Could you check a few things on this model? Use its own coordinates, in mm. Give positions to 0.01 mm unless a question says otherwise; leave off trailing zeros. Loops run counter-clockwise (first coordinate to the right, second up) from the corner with the lowest first, then second, coordinate; pieces in that order, holes last. Notation, with made-up numbers: M -33.75,-3.75 L 15.25,-3.75 A24 ccw 15.25,21.25 Z; hole C 47,14 d3. An arc over 180 degrees is marked long. Return JSON: item names as keys, results as strings. Group by question number.
1. If we section it at C-C (x = 3.83): Write out the boundary of the cut face in (y, z).
2. If we section it at B-B (x = 44.17): State how many separate pieces and enclosed holes the cut face has, plus the area to 3 significant figures.
3. Please list where these lines run through material, in increasing order: line 1 (Y direction, x = -44.17, z = 0.9) (3 decimals); line 2 (X direction, y = 120, z = 0.05); line 3 (X direction, y = 132, z = -0.7).
4. If we section it at D-D (y = 140): Write out the boundary of the cut face in (x, z).
5. If we section it at A-A (y = 90): Write out the boundary of the cut face in (x, z).
6. For pin 1 (4 mm diameter, centred on x = 44.17, y = 120, fed in from -Z), with a flat end and sliding along its axis, tell me the tip position at first contact or that it passes through.
```python
from build123d import *

# Parameters (mm, degrees)
STOCK_TORSO_REAR_PLATE_1_START       = -1.5875
STOCK_TORSO_REAR_PLATE_1_OUTLINE_W   = 96.34
STOCK_TORSO_REAR_PLATE_1_OUTLINE_H   = 125.5
STOCK_TORSO_REAR_PLATE_1_OUTLINE_R   = 1.45
STOCK_TORSO_REAR_PLATE_1_OUTLINE_W_2 = 3.4925
STOCK_TORSO_REAR_PLATE_1_OUTLINE_H_2 = 10.25
STOCK_TORSO_REAR_PLATE_1_DEPTH       = 3.175
MOVE_FACE1_BY                        = 0.5
CUT_EXTRUDE1_DEPTH                   = 158.576741701
CUT_EXTRUDE1_DEPTH_BACK              = 158.576741701
CUT_EXTRUDE2_DEPTH                   = 158.576741701
CUT_EXTRUDE2_DEPTH_BACK              = 158.576741701
SKETCH2_W                            = 25
SKETCH2_H                            = 62
FILLET1_R                            = 1
CUT_EXTRUDE3_DEPTH                   = 158.576741701
CUT_EXTRUDE3_DEPTH_BACK              = 158.576741701
FILLET2_R                            = 1


# Read off the part's stored shape, not the designer's step: Stock-torso_rear_plate-1
with BuildPart() as part:
    # Stock-torso_rear_plate-1 outline → Stock-torso_rear_plate-1 (new body)
    with BuildSketch(Plane.XY.offset(STOCK_TORSO_REAR_PLATE_1_START)):
        with Locations((0, 87.25)):
            Rectangle(STOCK_TORSO_REAR_PLATE_1_OUTLINE_W, STOCK_TORSO_REAR_PLATE_1_OUTLINE_H)
        with Locations((-44.17, 40)):
            Circle(STOCK_TORSO_REAR_PLATE_1_OUTLINE_R, mode=Mode.SUBTRACT)
        with BuildLine():
            Line((30, 34.5), (-30, 34.5))
            ThreePointArc((-30, 34.5), (-32.5, 37), (-30, 39.5))
            Line((-30, 39.5), (30, 39.5))
            ThreePointArc((30, 39.5), (32.5, 37), (30, 34.5))
        make_face(mode=Mode.SUBTRACT)
        with BuildLine():
            Line((30, 44.5), (-30, 44.5))
            ThreePointArc((-30, 44.5), (-32.5, 47), (-30, 49.5))
            Line((-30, 49.5), (30, 49.5))
            ThreePointArc((30, 49.5), (32.5, 47), (30, 44.5))
        make_face(mode=Mode.SUBTRACT)
        with Locations((44.17, 40)):
            Circle(STOCK_TORSO_REAR_PLATE_1_OUTLINE_R, mode=Mode.SUBTRACT)
        with BuildLine():
            ThreePointArc((-30, 54.5), (-32.5, 57), (-30, 59.5))
            Line((-30, 59.5), (30, 59.5))
            ThreePointArc((30, 59.5), (32.5, 57), (30, 54.5))
            Line((30, 54.5), (-30, 54.5))
        make_face(mode=Mode.SUBTRACT)
        with BuildLine():
            ThreePointArc((-30, 64.5), (-32.5, 67), (-30, 69.5))
            Line((-30, 69.5), (30, 69.5))
            ThreePointArc((30, 69.5), (32.5, 67), (30, 64.5))
            Line((30, 64.5), (-30, 64.5))
        make_face(mode=Mode.SUBTRACT)
        with Locations((-44.17, 120)):
            Circle(STOCK_TORSO_REAR_PLATE_1_OUTLINE_R, mode=Mode.SUBTRACT)
        with Locations((-44.17, 141)):
            Rectangle(STOCK_TORSO_REAR_PLATE_1_OUTLINE_W_2, STOCK_TORSO_REAR_PLATE_1_OUTLINE_H_2, mode=Mode.SUBTRACT)
        with Locations((44.17, 120)):
            Circle(STOCK_TORSO_REAR_PLATE_1_OUTLINE_R, mode=Mode.SUBTRACT)
        with Locations((44.17, 141)):
            Rectangle(STOCK_TORSO_REAR_PLATE_1_OUTLINE_W_2, STOCK_TORSO_REAR_PLATE_1_OUTLINE_H_2, mode=Mode.SUBTRACT)
    extrude(amount=STOCK_TORSO_REAR_PLATE_1_DEPTH)

    # Move Face1: a face moved inward by 0.5
    extrude(part.faces().sort_by_distance((0, 24.5, 0))[0], amount=MOVE_FACE1_BY, dir=(0, 1, 0), mode=Mode.SUBTRACT)

    # Sketch1 → Cut-Extrude1 (cut, two sides: drawn at the far end of the back side and taken through both)
    with BuildSketch(Plane.XY.offset(1.5875).offset(-CUT_EXTRUDE1_DEPTH_BACK)):
        with BuildLine():
            Line((1.83, 75), (1.83, 79))
            ThreePointArc((1.83, 79), (3.83, 81), (5.83, 79))
            Line((5.83, 79), (5.83, 75))
            ThreePointArc((5.83, 75), (3.83, 73), (1.83, 75))
        make_face()
        with BuildLine():
            Line((16.83, 75), (16.83, 79))
            ThreePointArc((16.83, 79), (18.83, 81), (20.83, 79))
            Line((20.83, 79), (20.83, 75))
            ThreePointArc((20.83, 75), (18.83, 73), (16.83, 75))
        make_face()
    extrude(amount=CUT_EXTRUDE1_DEPTH + CUT_EXTRUDE1_DEPTH_BACK, mode=Mode.SUBTRACT)

    # Sketch2 → Cut-Extrude2 (cut, two sides: drawn at the far end of the back side and taken through both)
    with BuildSketch(Plane(origin=(0, 0, -1.5875), x_dir=(-1, 0, 0), z_dir=(0, 0, -1)).offset(-CUT_EXTRUDE2_DEPTH_BACK)):
        with Locations((-23.67, 114)):
            Rectangle(SKETCH2_W, SKETCH2_H)
    extrude(amount=CUT_EXTRUDE2_DEPTH + CUT_EXTRUDE2_DEPTH_BACK, mode=Mode.SUBTRACT)

    # Fillet1
    fillet1_edges = [part.edges().sort_by_distance(p)[0] for p in [
        (36.17, 83, 0),
        (36.17, 145, 0),
        (11.17, 145, 0),
        (11.17, 83, 0),
    ]]
    fillet(fillet1_edges, radius=FILLET1_R)

    # Sketch3 → Cut-Extrude3 (cut, two sides: drawn at the far end of the back side and taken through both)
    with BuildSketch(Plane(origin=(0, 0, -1.5875), x_dir=(-1, 0, 0), z_dir=(0, 0, -1)).offset(-CUT_EXTRUDE3_DEPTH_BACK)):
        with BuildLine():
            Line((0, 92.5), (30, 92.5))
            ThreePointArc((30, 92.5), (32.5, 90), (30, 87.5))
            Line((30, 87.5), (0, 87.5))
            ThreePointArc((0, 87.5), (-2.5, 90), (0, 92.5))
        make_face()
        with BuildLine():
            Line((0, 102.5), (30, 102.5))
            ThreePointArc((30, 102.5), (32.5, 100), (30, 97.5))
            Line((30, 97.5), (0, 97.5))
            ThreePointArc((0, 97.5), (-2.5, 100), (0, 102.5))
        make_face()
        with BuildLine():
            Line((0, 112.5), (30, 112.5))
            ThreePointArc((30, 112.5), (32.5, 110), (30, 107.5))
            Line((30, 107.5), (0, 107.5))
            ThreePointArc((0, 107.5), (-2.5, 110), (0, 112.5))
        make_face()
        with BuildLine():
            Line((0, 122.5), (30, 122.5))
            ThreePointArc((30, 122.5), (32.5, 120), (30, 117.5))
            Line((30, 117.5), (0, 117.5))
            ThreePointArc((0, 117.5), (-2.5, 120), (0, 122.5))
        make_face()
        with BuildLine():
            Line((0, 132.5), (30, 132.5))
            ThreePointArc((30, 132.5), (32.5, 130), (30, 127.5))
            Line((30, 127.5), (0, 127.5))
            ThreePointArc((0, 127.5), (-2.5, 130), (0, 132.5))
        make_face()
        with BuildLine():
            Line((0, 142.5), (30, 142.5))
            ThreePointArc((30, 142.5), (32.5, 140), (30, 137.5))
            Line((30, 137.5), (0, 137.5))
            ThreePointArc((0, 137.5), (-2.5, 140), (0, 142.5))
        make_face()
    extrude(amount=CUT_EXTRUDE3_DEPTH + CUT_EXTRUDE3_DEPTH_BACK, mode=Mode.SUBTRACT)

    # Fillet2
    fillet2_edges = [part.edges().sort_by_distance(p)[0] for p in [
        (48.17, 25, 0),
        (-48.17, 25, 0),
        (48.17, 150, 0),
        (-48.17, 150, 0),
    ]]
    fillet(fillet2_edges, radius=FILLET2_R)


solid = part.part
```
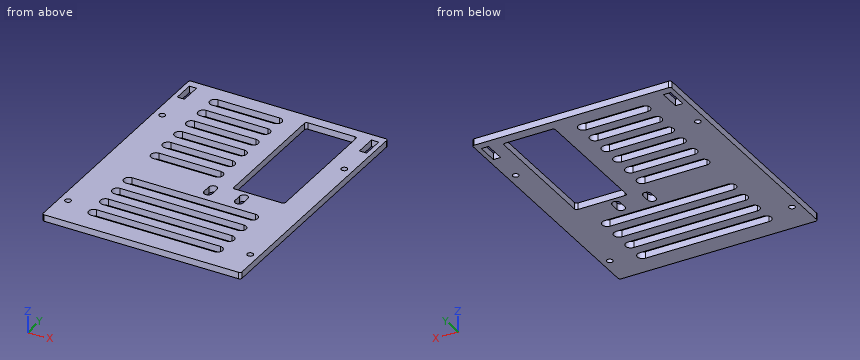
Answer:
{
 "1": {"outline": "M 25,-1.59 L 34.5,-1.59 L 34.5,1.59 L 25,1.59 Z; M 39.5,-1.59 L 44.5,-1.59 L 44.5,1.59 L 39.5,1.59 Z; M 49.5,-1.59 L 54.5,-1.59 L 54.5,1.59 L 49.5,1.59 Z; M 59.5,-1.59 L 64.5,-1.59 L 64.5,1.59 L 59.5,1.59 Z; M 69.5,-1.59 L 73,-1.59 L 73,1.59 L 69.5,1.59 Z; M 81,-1.59 L 150,-1.59 L 150,1.59 L 81,1.59 Z"},
 "2": {"separate pieces": "4", "enclosed holes": "0", "area": "346 mm²"},
 "3": {"line 1": "y = 25 to 38.55, 41.45 to 118.55, 121.45 to 135.875, 146.125 to 150", "line 2": "x = -48.17 to -45.62, -42.72 to -32.5, 2.5 to 11.17, 36.17 to 42.72, 45.62 to 48.17", "line 3": "x = -48.17 to -31.5, 1.5 to 11.17, 36.17 to 48.17"},
 "4": {"outline": "M -48.17,-1.59 L -45.92,-1.59 L -45.92,1.59 L -48.17,1.59 Z; M -42.42,-1.59 L -32.5,-1.59 L -32.5,1.59 L -42.42,1.59 Z; M 2.5,-1.59 L 11.17,-1.59 L 11.17,1.59 L 2.5,1.59 Z; M 36.17,-1.59 L 42.42,-1.59 L 42.42,1.59 L 36.17,1.59 Z; M 45.92,-1.59 L 48.17,-1.59 L 48.17,1.59 L 45.92,1.59 Z"},
 "5": {"outline": "M -48.17,-1.59 L -32.5,-1.59 L -32.5,1.59 L -48.17,1.59 Z; M 2.5,-1.59 L 11.17,-1.59 L 11.17,1.59 L 2.5,1.59 Z; M 36.17,-1.59 L 48.17,-1.59 L 48.17,1.59 L 36.17,1.59 Z"},
 "6": {"pin 1": "stops at z = -1.59"}
}
